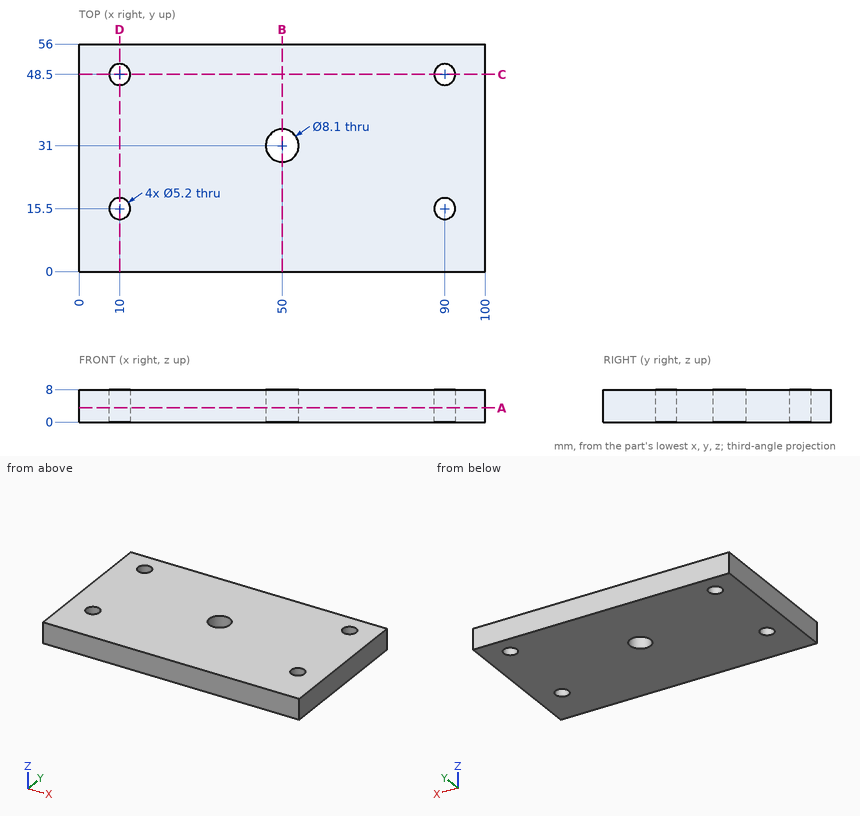
Could you check a few things on this drawing? It's one solid part, dimensions in mm from its lowest x, y, z. Coordinates: 2 decimals unless noted, no trailing zeros. Order: outer loops, then holes, each group sorted by start corner. A loop starts at its lowest first (then second) coordinate and runs counter-clockwise, first axis right, second up. Notation, with made-up numbers: (-33.75, 12.5) - (15.25, 12.5) arc R13 ccw to (15.25, 34.5) - close; hole circle Ø5 at (-26, -25). An arc over 180 degrees is marked (long way). Answer as a JSON object with one key per item and string values. Group by question number.
Q1. Imagine slicing it at D-D (x = 10). Please give me the cut outline in (y, z), and give its area (3 significant figures).
Q2. I need wall thicknesses on line 1 (Y direction, x = 90, z = 4.75); line 2 (Y direction, x = 50, z = 5.75); line 3 (Y direction, x = 12, z = 1.25). Which ranges of each line are inside material? Lowest first, please. Write a range as from..to.
Q3. Imagine slicing it at A-A (z = 3.5). Please give me the cut outline in (x, y).
Q4. Imagine slicing it at B-B (x = 50). Please give me the cut outline in (y, z).
Q5. Imagine slicing it at C-C (y = 48.5). Please give me the cut outline in (x, z).
Determined:
{
 "1": {"outline": "(0, 0) - (12.9, 0) - (12.9, 8) - (0, 8) - close; (18.1, 0) - (45.9, 0) - (45.9, 8) - (18.1, 8) - close; (51.1, 0) - (56, 0) - (56, 8) - (51.1, 8) - close", "area": "365 mm2"},
 "2": {"line 1": "y = 0..12.9, 18.1..45.9, 51.1..56", "line 2": "y = 0..26.95, 35.05..56", "line 3": "y = 0..13.84, 17.16..46.84, 50.16..56"},
 "3": {"outline": "(0, 0) - (100, 0) - (100, 56) - (0, 56) - close; hole circle Ø5.2 at (10, 15.5); hole circle Ø5.2 at (10, 48.5); hole circle Ø8.1 at (50, 31); hole circle Ø5.2 at (90, 15.5); hole circle Ø5.2 at (90, 48.5)"},
 "4": {"outline": "(0, 0) - (26.95, 0) - (26.95, 8) - (0, 8) - close; (35.05, 0) - (56, 0) - (56, 8) - (35.05, 8) - close"},
 "5": {"outline": "(0, 0) - (7.4, 0) - (7.4, 8) - (0, 8) - close; (12.6, 0) - (87.4, 0) - (87.4, 8) - (12.6, 8) - close; (92.6, 0) - (100, 0) - (100, 8) - (92.6, 8) - close"}
}
